Read the model definition and answer for the solid it produces. Units are mm, in the model's axes. Face numbers are marked on the shaded views. A direction names the side the tool comes from. Give positions to 0.01 mm unless a question says otherwise; leave off trailing zeros. Write each loop counter-clockwise with the first axis right and the second up, starting at its lowest first coordinate (ties: lowest second). Pieces come first, ordered by that corner, then holes. Notation, with made-up numbers: (-0.5, -39.75) -> (48.5, -39.75) arc R27 cw to (48.5, -18.75) -> close; hole circle Ø2 at (-25, 66.25). An arc over 180 degrees is marked (long way). Write item = value, one per line.
from build123d import *

# Parameters (mm, degrees)
F0_R     = 39.6875
F0_R_2   = 9.652
F1_DEPTH = 19.05
F2_R     = 15.8369
F2_R_2   = 9.652
F3_DEPTH = 48.26
F4_R     = 2.4645418127
F5_DEPTH = 12.7
F7_DEPTH = 45.72


with BuildPart() as f1:
    # F0 (on Top) → F1 (new body)
    with BuildSketch(Plane.XY):
        Circle(F0_R)
        Circle(F0_R_2, mode=Mode.SUBTRACT)
    extrude(amount=F1_DEPTH)

    # F2 (on face) → F3 (join)
    with BuildSketch(Plane.XY.offset(19.05)):
        Circle(F2_R)
        Circle(F2_R_2, mode=Mode.SUBTRACT)
    extrude(amount=F3_DEPTH)

    # F4 (on face) → F5 (cut)
    with BuildSketch(Plane(origin=(0, 0, 0), x_dir=(1, 0, 0), z_dir=(0, 0, -1))):
        with Locations((-31.75, 0)):
            Circle(F4_R)
        with Locations((0, -31.75)):
            Circle(F4_R)
        with Locations((0, 31.75)):
            Circle(F4_R)
        with Locations((31.75, 0)):
            Circle(F4_R)
    extrude(amount=-F5_DEPTH, mode=Mode.SUBTRACT)

    # F6 (on face) → F7 (cut)
    with BuildSketch(Plane.XY.offset(67.31)):
        with BuildLine():
            Line((15.757133158, -1.5875), (25.4, -1.5875))
            Line((25.4, -1.5875), (25.4, 1.5875))
            Line((25.4, 1.5875), (15.757133158, 1.5875))
            ThreePointArc((15.757133158, 1.5875), (15.8169457184, 0.7947513761), (15.8369, 0))
            ThreePointArc((15.8369, 0), (15.8169457184, -0.7947513761), (15.757133158, -1.5875))
        make_face()
        with BuildLine():
            Line((9.5205539623, -1.5875), (15.757133158, -1.5875))
            ThreePointArc((15.757133158, -1.5875), (15.8169457184, -0.7947513761), (15.8369, 0))
            ThreePointArc((15.8369, 0), (15.8169457184, 0.7947513761), (15.757133158, 1.5875))
            Line((15.757133158, 1.5875), (9.5205539623, 1.5875))
            ThreePointArc((9.5205539623, 1.5875), (9.6190823586, 0.7964663067), (9.652, 0))
            ThreePointArc((9.652, 0), (9.6190823586, -0.7964663067), (9.5205539623, -1.5875))
        make_face()
        with BuildLine():
            ThreePointArc((-15.757133158, 1.5875), (-15.8369, 0), (-15.757133158, -1.5875))
            Line((-15.757133158, -1.5875), (-9.5205539623, -1.5875))
            ThreePointArc((-9.5205539623, -1.5875), (-9.652, 0), (-9.5205539623, 1.5875))
            Line((-9.5205539623, 1.5875), (-15.757133158, 1.5875))
        make_face()
        with BuildLine():
            Line((-25.4, -1.5875), (-15.757133158, -1.5875))
            ThreePointArc((-15.757133158, -1.5875), (-15.8369, 0), (-15.757133158, 1.5875))
            Line((-15.757133158, 1.5875), (-25.4, 1.5875))
            Line((-25.4, 1.5875), (-25.4, -1.5875))
        make_face()
    extrude(amount=-F7_DEPTH, mode=Mode.SUBTRACT)


solid = f1.part
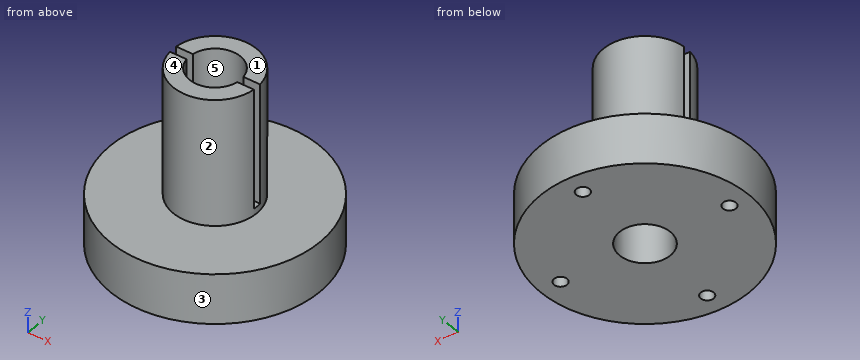
(1) Consider L1, parallel to X at y = 1.5, z = 6; L2, parallel to Y at x = 0, z = 40; L3, parallel to Z at x = 24.5, y = -19. Determine where each line is inside the solid, lowest interval first.
Checks:
L1 = -39.66 to -33.71, -29.79 to -9.53, 9.53 to 29.79, 33.71 to 39.66
L2 = -15.84 to -9.65, 9.65 to 15.84
L3 = 0 to 19.05
(2) The part is cut by section A-A on z = 37.5. Determine the outline of the cut face in (x, y).
Checks:
outline = (-15.76, -1.59) arc R15.84 ccw to (15.76, -1.59) -> (9.52, -1.59) arc R9.65 cw to (-9.52, -1.59) -> close; (-15.76, 1.59) -> (-9.52, 1.59) arc R9.65 cw to (9.52, 1.59) -> (15.76, 1.59) arc R15.84 ccw to start
(3) The part is cut by section B-B on y = 0. Determine the outline of the cut face in (x, z), plus the area to 3 significant figures.
Checks:
outline = (-39.69, 0) -> (-34.21, 0) -> (-34.21, 12.7) -> (-29.29, 12.7) -> (-29.29, 0) -> (-9.65, 0) -> (-9.65, 21.59) -> (-15.84, 21.59) -> (-15.84, 19.05) -> (-39.69, 19.05) -> close; (9.65, 0) -> (29.29, 0) -> (29.29, 12.7) -> (34.21, 12.7) -> (34.21, 0) -> (39.69, 0) -> (39.69, 19.05) -> (15.84, 19.05) -> (15.84, 21.59) -> (9.65, 21.59) -> close
area = 1,050 mm²
(4) The part is cut by section C-C on z = 6. Count the separate pieces of the cut face and the enclosed holes in it, plus the area to 3 significant figures.
Checks:
separate_pieces = 1
enclosed_holes = 5
area = 4,580 mm²
(5) Given P1, Ø5.5, axis at x = 31.75, y = 0, coming from the +Z side; P2, Ø4, axis at x = -20.5, z = 19, coming from the +Y side; P3, Ø5, axis at x = -12, z = 55.5, coming from the +Y side, each flat-ended and moving along its own axis, determine where each tip first touches the part or whether it passes through.
Checks:
P1 = 19.05
P2 = 35.11
P3 = 12.67
(6) The part is cut by section D-D on x = 7. Determine the outline of the cut face in (y, z), plus the area to 3 significant figures.
Checks:
outline = (-39.07, 0) -> (-6.65, 0) -> (-6.65, 67.31) -> (-14.21, 67.31) -> (-14.21, 19.05) -> (-39.07, 19.05) -> close; (6.65, 0) -> (39.07, 0) -> (39.07, 19.05) -> (14.21, 19.05) -> (14.21, 67.31) -> (6.65, 67.31) -> close
area = 1,960 mm²
(7) A tool of negligible diameter and unlimited length cuts with its end or side. For the marked faces 1 and 2, from which of +Z, -Z, +X, -X, +Y, -Y can it reach the whole face along a straight path? Write none if from no direction.
Checks:
face_1 = +Z, +X, -X, +Y, -Y
face_2 = +Z
(8) For a pull along Y with two mould halves and no side action, classify the marked faces 3, 4 and 5 as released by +Y, released by -Y, zero draft, split by the parting line, or undercut.
Checks:
face_3 = split by the parting line
face_4 = zero draft
face_5 = undercut
